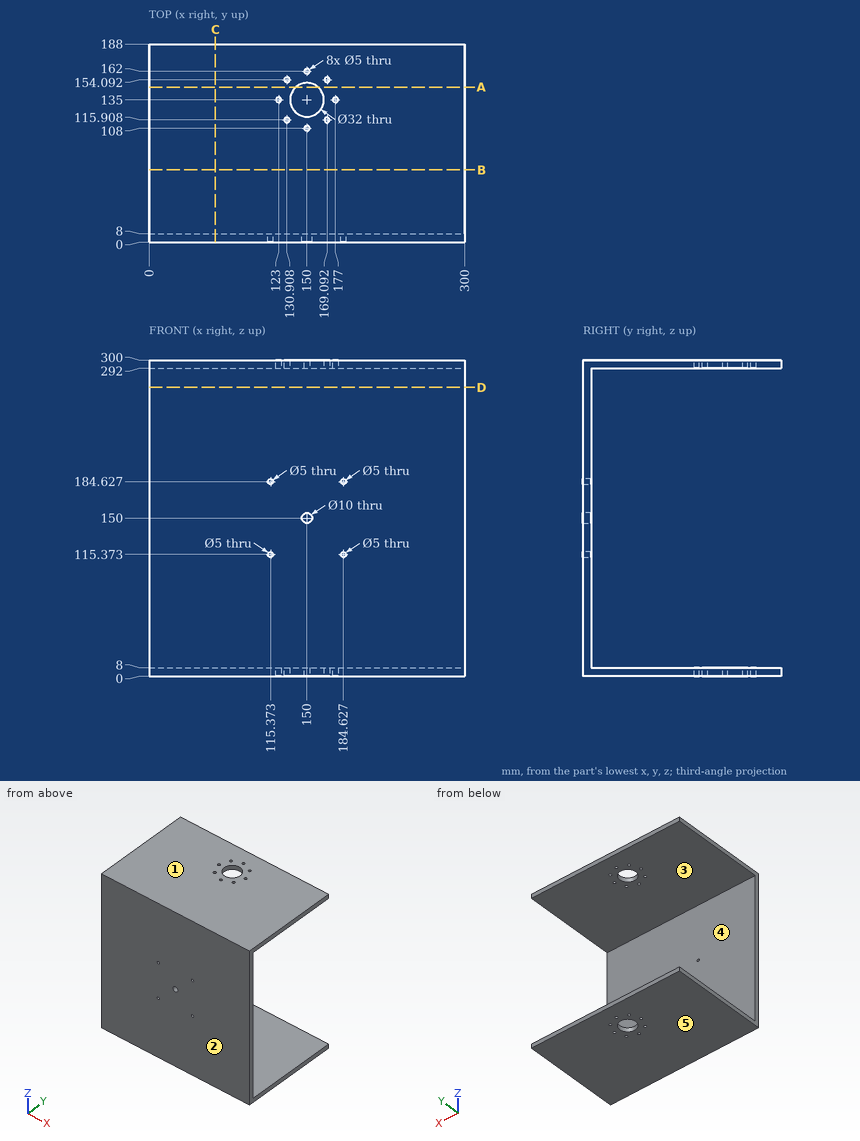
Input: dimensioned drawing with shaded views. Units: mm. Origin: part minimum x, y, z. A direction names the side the tool comes from. Give positions to 0.01 mm unless a question says otherwise; leave off trailing zeros. Order: outer loops, then holes, each group sorted by start corner. A loop starts at its lowest first (then second) coordinate and runs counter-clockwise, first axis right, second up.
(1) Pull-direction query (Z, two-part tool) for the marked faces 1, 2 and 3; classes: +Z half, -Z half, draft (parallel to the pull), parting line (faces both ways), or undercut.
(2) Access query for the marked faces 4 and 5. Directions: +Z, -Z, +X, -X, +Y, -Y. A direction counts if a zero-diameter tool reaches every point of the face in a straight line with its end or side. Return the directions, or none.
(3) Contact query for a flat-ended pin moving along its axis: P1, Ø6, axis at x = 255.5, z = 33.5, coming from the +Y side. Output: stop coordinate, or through.
(4) Section query A-A (y = 147). Return the cut outline in (x, z), plus the area to 3 significant figures.
(5) Section query D-D (z = 274). Return the cut outline in (x, y).
(6) Section query B-B (y = 68.5). Return the cut outline in (x, z), plus the area to 3 significant figures.
(7) Section query C-C (x = 63). Return the cut outline in (y, z).
(8) Material intervals for line 1 along Y through (x, z) = (150, 5); line 2 along Z through (x, y) = (140, 168); line 3 along X through (y, z) = (162, 295), sorted ascending.
Outcome:
1. face 1: +Z half
1. face 2: draft
1. face 3: undercut
2. face 4: +X, -X, +Y
2. face 5: -Z, +X, -X, +Y, -Y
3. P1: stops at y = 8
4. outline: (0, 0) - (139.42, 0) - (139.42, 8) - (0, 8) - close; (0, 292) - (139.42, 292) - (139.42, 300) - (0, 300) - close; (160.58, 0) - (300, 0) - (300, 8) - (160.58, 8) - close; (160.58, 292) - (300, 292) - (300, 300) - (160.58, 300) - close
4. area: 4,460 mm2
5. outline: (0, 0) - (300, 0) - (300, 8) - (0, 8) - close
6. outline: (0, 0) - (300, 0) - (300, 8) - (0, 8) - close; (0, 292) - (300, 292) - (300, 300) - (0, 300) - close
6. area: 4,800 mm2
7. outline: (0, 0) - (188, 0) - (188, 8) - (8, 8) - (8, 292) - (188, 292) - (188, 300) - (0, 300) - close
8. line 1: y = 0 to 105.5, 110.5 to 119, 151 to 159.5, 164.5 to 188
8. line 2: z = 0 to 8, 292 to 300
8. line 3: x = 0 to 147.5, 152.5 to 300
